Build history of the part. All positions in model axes, mm. Give positions to 0.01 mm unless a question says otherwise; leave off trailing zeros. Order: outer loops, then holes, each group sorted by start corner. A loop starts at its lowest first (then second) coordinate and runs counter-clockwise, first axis right, second up. Notation, with made-up numbers: (-27, 57.5) - (22, 57.5) arc R24 cw to (22, 92.5) - close; hole circle Ø10 at (59, 79). An arc over 180 degrees is marked (long way). Use a Markdown table: item, result.
from build123d import *

# Parameters (mm, degrees)
BOSS_EXTRU_1_DEPTH                             = 4
FRAISAGE_POUR_VIS_T_TE_FRAIS_E_M31_D           = 3.4
FRAISAGE_POUR_VIS_T_TE_FRAIS_E_M31_CSINK_D     = 6.3
FRAISAGE_POUR_VIS_T_TE_FRAIS_E_M31_CSINK_ANGLE = 90
CONG_1_R                                       = 5
D_GAGEMENT_M81_D                               = 9
CONG_2_R                                       = 3
CHANFREIN1_SIZE                                = 0.5
CHANFREIN2_SIZE                                = 0.5


with BuildPart() as part:
    # Esquisse1 → Boss.-Extru.1 (new body)
    with BuildSketch(Plane.XY):
        Polygon((0, 77), (4.5, 77), (4.5, 23), (0, 23), (0, 0), (-45, 0), (-45, 23), (-49.5, 23), (-49.5, 77), (-45, 77), (-45, 100), (0, 100), align=None)
    extrude(amount=BOSS_EXTRU_1_DEPTH)

    # Fraisage pour vis à tête fraisée M31 (through all)
    with Locations(Plane.XY.offset(4)):
        with Locations((-44.5, 72), (-0.5, 72), (-0.5, 28), (-44.5, 28)):
            CounterSinkHole(FRAISAGE_POUR_VIS_T_TE_FRAIS_E_M31_D / 2, FRAISAGE_POUR_VIS_T_TE_FRAIS_E_M31_CSINK_D / 2, counter_sink_angle=FRAISAGE_POUR_VIS_T_TE_FRAIS_E_M31_CSINK_ANGLE)

    # Congé1
    # the kernel refuses this fillet: 5 mm, written as the material it takes off along each edge
    with BuildSketch(Plane(origin=(-49.5, 23, -12.437342964), x_dir=(0, 1, 0), z_dir=(0, 0, 1))) as cong_1_piece_1:
        with BuildLine():
            CenterArc((4.974937186, -5), CONG_1_R, 90, 84.260829523)
            Line((0, -4.5), (-0.099498744, -4.49))
            ThreePointArc((-0.099498744, -4.49), (-0.1, -2.25), (-0.1, 0))
            Line((-0.1, 0), (0, 0.1))
            Line((0, 0.1), (4.974937186, 0.1))
            Line((4.974937186, 0.1), (4.974937186, 0))
        make_face()
    extrude(amount=28.874685928, mode=Mode.SUBTRACT)
    with BuildSketch(Plane(origin=(-49.5, 77, -12.437342964), x_dir=(1, 0, 0), z_dir=(0, 0, 1)), Plane(origin=(4.5, 23, -12.437342964), x_dir=(-1, 0, 0), z_dir=(0, 0, 1))) as cong_1_piece_2:
        with BuildLine():
            CenterArc((5, -4.974937186), CONG_1_R, 95.739170477, 84.260829523)
            Line((0, -4.974937186), (-0.1, -4.974937186))
            Line((-0.1, -4.974937186), (-0.1, 0))
            Line((-0.1, 0), (0, 0.1))
            ThreePointArc((0, 0.1), (2.25, 0.1), (4.49, 0.099498744))
            Line((4.49, 0.099498744), (4.5, 0))
        make_face()
    extrude(amount=28.874685928, mode=Mode.SUBTRACT)
    with BuildSketch(Plane(origin=(4.5, 77, -12.437342964), x_dir=(-1, 0, 0), z_dir=(0, 0, 1))) as cong_1_piece_3:
        with BuildLine():
            CenterArc((5, 4.974937186), CONG_1_R, 180, 84.260829523)
            Line((0, 4.974937186), (-0.1, 4.974937186))
            Line((-0.1, 4.974937186), (-0.1, 0))
            Line((-0.1, 0), (0, -0.1))
            ThreePointArc((0, -0.1), (2.25, -0.1), (4.49, -0.099498744))
            Line((4.49, -0.099498744), (4.5, 0))
        make_face()
    extrude(amount=28.874685928, mode=Mode.SUBTRACT)

    # Dégagement M81 (through all)
    with Locations(Plane.XY.offset(4)):
        with Locations((-22.5, 88.5), (-22.5, 11.5)):
            Hole(D_GAGEMENT_M81_D / 2)

    # Congé2
    cong_2_edges = [part.edges().sort_by_distance(p)[0] for p in [
        (-45, 100, 2),
        (0, 100, 2),
        (0, 0, 2),
        (-45, 0, 2),
    ]]
    fillet(cong_2_edges, radius=CONG_2_R)

    # Chanfrein1
    chanfrein1_edges = [part.edges().sort_by_distance(p)[0] for p in [
        (0, 87, 0),
        (-45, 13, 0),
        (-49.5, 50, 0),
        (4.5, 50, 0),
        (3.208099244, 24.620835219, 0),
        (-48.208099244, 75.379164781, 0),
        (-48.208099244, 24.620835219, 0),
        (3.208099244, 75.379164781, 0),
        (4.5, 50, 4),
        (3.208099244, 24.620835219, 4),
        (3.208099244, 75.379164781, 4),
        (0, 13, 0),
        (-22.5, 0, 0),
        (-45, 87, 0),
        (-22.5, 100, 0),
        (-0.878679656, 99.121320344, 0),
        (-44.121320344, 99.121320344, 0),
        (-44.121320344, 0.878679656, 0),
        (-0.878679656, 0.878679656, 0),
    ]]
    chamfer(chanfrein1_edges, length=CHANFREIN1_SIZE)

    # Chanfrein2
    chanfrein2_edges = [part.edges().sort_by_distance(p)[0] for p in [
        (0, 86.748599385, 4),
        (-0.878679656, 99.121320344, 4),
        (-22.5, 100, 4),
        (-44.121320344, 99.121320344, 4),
        (-45, 87, 4),
        (-45, 13, 4),
        (-44.121320344, 0.878679656, 4),
        (-22.5, 0, 4),
        (-0.878679656, 0.878679656, 4),
        (0, 13.251400615, 4),
        (-48.208099244, 75.379164781, 4),
        (-48.208099244, 24.620835219, 4),
        (-49.5, 50, 4),
    ]]
    chamfer(chanfrein2_edges, length=CHANFREIN2_SIZE)


solid = part.part
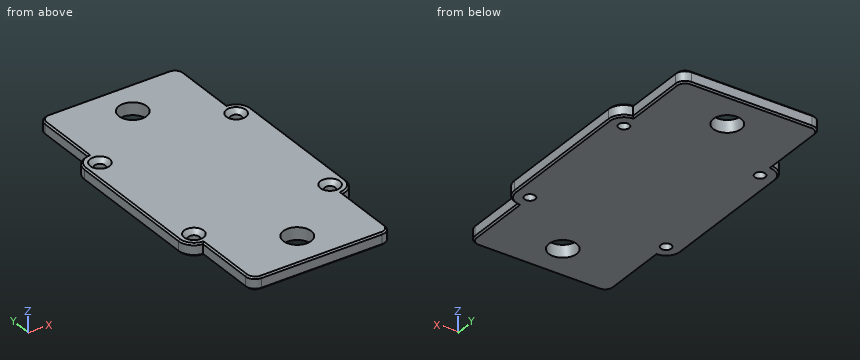
1) Slice it at C-C (x = -22.5). Write the cut outline in (y, z).
Computed:
| item | result |
|---|---|
| outline | (0, 0.5) - (0.5, 0) - (7, 0) - (7, 4) - (0.5, 4) - (0, 3.5) - close; (16, 0) - (84, 0) - (84, 4) - (16, 4) - close; (93, 0) - (99.5, 0) - (100, 0.5) - (100, 3.5) - (99.5, 4) - (93, 4) - close |
2) Pin check, flat tips, straight feed: P1, Ø4.5, axis at x = -0.5, y = 72, coming from the +Z side; P2, Ø1.5, axis at y = 88.5, z = 1, coming from the -X side; P3, Ø3, axis at x = -13, y = 47.5, coming from the -Z side; P4, Ø0.9, axis at y = 91.5, z = 2, coming from the +X side. Stop position of each tip, or through.
Computed:
| item | result |
|---|---|
| P1 | stops at z = 3.1 |
| P2 | stops at x = -45 |
| P3 | stops at z = 0 |
| P4 | stops at x = 0 |
3) Slice it at A-A (z = 1.6). Write the cut outline in (x, y).
Computed:
| item | result |
|---|---|
| outline | (-49.5, 27.97) arc R5 ccw to (-45, 23) - (-45, 3) arc R3 ccw to (-42, 0) - (-3, 0) arc R3 ccw to (0, 3) - (0, 23) arc R5 ccw to (4.5, 27.97) - (4.5, 72.03) arc R5 ccw to (0, 77) - (0, 97) arc R3 ccw to (-3, 100) - (-42, 100) arc R3 ccw to (-45, 97) - (-45, 77) arc R5 ccw to (-49.5, 72.03) - close; hole circle Ø3.4 at (-44.5, 28); hole circle Ø3.4 at (-44.5, 72); hole circle Ø9 at (-22.5, 11.5); hole circle Ø9 at (-22.5, 88.5); hole circle Ø3.4 at (-0.5, 28); hole circle Ø3.4 at (-0.5, 72) |
4) Wall check: line 1 (X direction, y = 72, z = 1.7); line 2 (Y direction, x = -22.5, z = 3.05); line 3 (X direction, y = 72, z = 0.3). Give the ranges that are in metal, low to high. Write a range as from..to.
Computed:
| item | result |
|---|---|
| line 1 | x = -49.5..-46.2, -42.8..-2.2, 1.2..4.5 |
| line 2 | y = 0..7, 16..84, 93..100 |
| line 3 | x = -49.3..-46.2, -42.8..-2.2, 1.2..4.3 |
5) Slice it at B-B (y = 88.5). Write the cut outline in (x, z), and give its area (4 significant figures).
Computed:
| item | result |
|---|---|
| outline | (-45, 0.5) - (-44.5, 0) - (-27, 0) - (-27, 4) - (-44.5, 4) - (-45, 3.5) - close; (-18, 0) - (-0.5, 0) - (0, 0.5) - (0, 3.5) - (-0.5, 4) - (-18, 4) - close |
| area | 143.5 mm² |
